CAD build for the part. Positions are in the model's coordinates, mm. Round coordinates to 2 decimals unless told otherwise and drop trailing zeros. Put each result on its own line as item: value.
```python
from build123d import *

# Parameters (mm, degrees)
SKETCH3_R           = 4.445
SKETCH3_R_2         = 1.2573
BOSS_EXTRUDE1_DEPTH = 1.778
BOSS_EXTRUDE2_DEPTH = 1.778
CIRPATTERN1_COUNT   = 5


with BuildPart() as part:
    # Sketch1 → Revolve1 (revolve)
    with BuildSketch(Plane.XY):
        with BuildLine():
            Line((-1.778, 49.53), (1.778, 49.53))
            Line((1.778, 49.53), (1.778, 54.61))
            ThreePointArc((1.778, 54.61), (0, 52.832), (-1.778, 54.61))
            Line((-1.778, 54.61), (-1.778, 49.53))
        make_face()
    revolve(axis=Axis((0, 0, 0), (-1, 0, 0)))



with BuildPart() as body_2:
    # Sketch3 → Boss-Extrude1 (new body, symmetric)
    with BuildSketch(Plane(origin=(0, 0, 0), x_dir=(0, 0, -1), z_dir=(1, 0, 0))):
        Circle(SKETCH3_R)
        Circle(SKETCH3_R_2, mode=Mode.SUBTRACT)
    extrude(amount=BOSS_EXTRUDE1_DEPTH, both=True)


with BuildPart() as part_1:
    add(part.part)

    add(body_2.part)  # Boss-Extrude2 merges body 2
    # Sketch4 → Boss-Extrude2 (add, symmetric)
    with BuildSketch(Plane(origin=(0, 0, 0), x_dir=(0, 0, -1), z_dir=(1, 0, 0))):
        with BuildLine():
            add(Edge.make_bspline(
                [(4.236760603, 1.34457599), (-0.842126183, 33.70804678), (-7.397626382, 44.22942933), (-18.096543838, 46.105704648)],
                knots=[0.007889083, 0.007889083, 0.007889083, 0.007889083, 0.582841342, 0.582841342, 0.582841342, 0.582841342], degree=3))
            ThreePointArc((-18.096543838, 46.105704648), (-24.282655216, 43.169127344), (-30.004622023, 39.407404853))
            add(Edge.make_bspline(
                [(2.269041799, 3.822234204), (-8.811754066, 30.630525708), (-30.004622023, 39.407404853)],
                knots=[0, 0, 0, 0.677750608, 0.677750608, 0.677750608], degree=2))
            ThreePointArc((2.269041799, 3.822234204), (3.480813667, 2.764409742), (4.236760603, 1.34457599))
        make_face()
    boss_extrude2 = extrude(amount=BOSS_EXTRUDE2_DEPTH, both=True)

    # CirPattern1: Boss-Extrude2 ×5 about axis
    cirpattern1_axis = Axis((0, 0, 0), (1, 0, 0))
    for i in range(1, CIRPATTERN1_COUNT):
        add(boss_extrude2.rotate(cirpattern1_axis, i * 360 / CIRPATTERN1_COUNT))


solid = part_1.part
```
Item 1: Pin check, flat tips, straight feed: P1, Ø1.5, axis at x = 0.5, z = 21, coming from the -Y side; P2, Ø1.5, axis at x = -0.5, y = -27, coming from the +Z side; P3, Ø1, axis at x = 0, z = -8, coming from the +Y side. Stop position of each tip, or through.
Answers below:
P1: y = -49.1
P2: z = 46.12
P3: y = 52.31
Item 2: Probe line 1 along Z through (x, y) = (-0.4, 12); line 2 along Y through (x, z) = (0.75, 37); line 3 along Y through (x, z) = (-0.1, -20). List the from-to ranges inside material, lowest first. Write a range as [from, to].
Answers below:
line 1: [-51.5, -48.05], [-28.15, -16.78], [-2.35, 1.57], [48.05, 51.5]
line 2: [-37.94, -32.93], [-7.57, 5.86], [32.93, 37.94]
line 3: [-48.9, -45.31], [-22.99, -13.34], [6.16, 16.63], [45.31, 48.9]
Item 3: Band-saw the part on A-A on y = 29. State how many separate pieces and enclosed holes the cut face has, and give its area (3 significant figures).
Answers below:
separate pieces: 4
enclosed holes: 0
area: 119 mm²
Item 4: Mould opens along Z. For faces 1 (the flat face through (-1.778, 4, 4)), 2 (the cylindrical face through (0.02, -43, -24.58)), 3 (the cylindrical face through (0.02, 10.09, -48.49)) say: pulls with the +Z half, pulls with the -Z half, needs draft (parallel to the pull), parting line crosses it, or undercut.
Answers below:
face 1: needs draft
face 2: undercut
face 3: undercut
